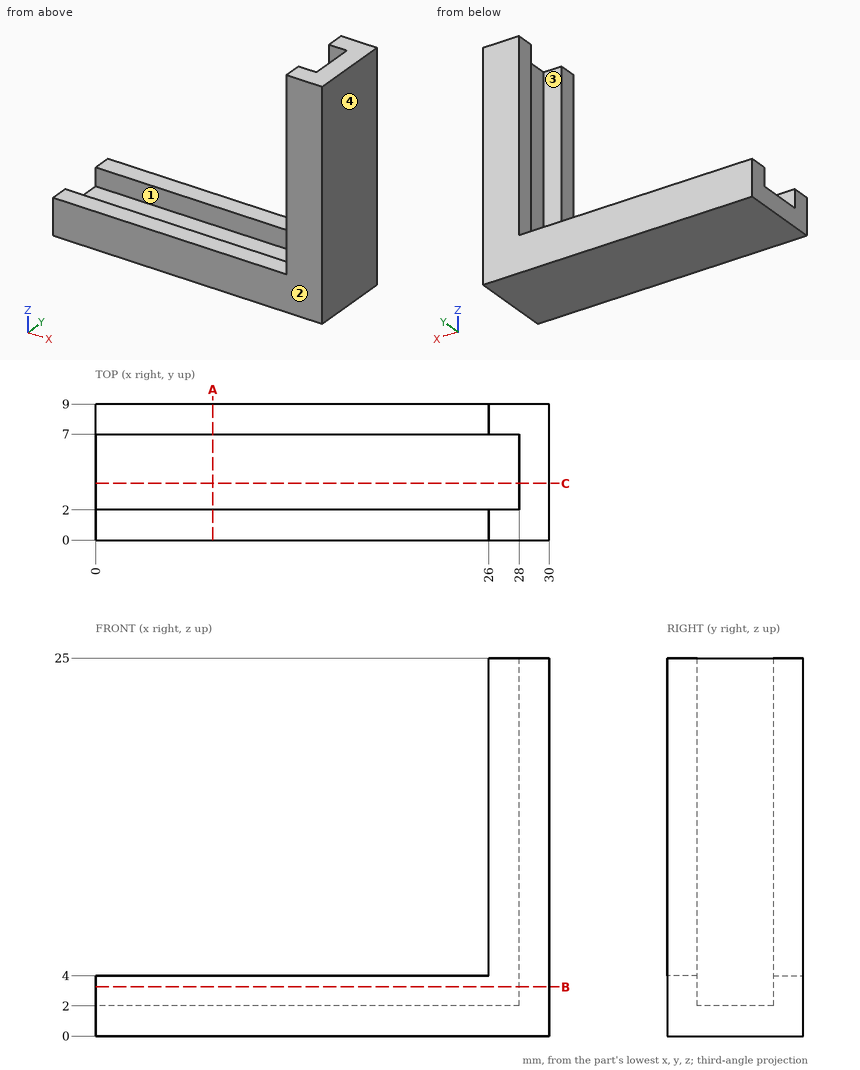
Could you check a few things on this drawing? It's one solid part, dimensions in mm from its lowest x, y, z. Coordinates: 2 decimals unless noted, no trailing zeros. Write each loop counter-clockwise with the first axis right and the second up, starting at its lowest first coordinate (ties: lowest second). Pieces come first, ordered by that corner, then holes. Notation, with made-up numbers: (78.5, -13.75) - (108.5, -13.75) arc R20 cw to (108.5, 24.25) - close; hole circle Ø4 at (3, -6.5). An arc over 180 degrees is marked (long way). Use one line per item in the form item = value.
1) Suppose I cut it at B-B, the plane z = 3.25. Write out the boundary of the cut face in (x, y), plus the area to 3 significant figures.
Solved:
outline = (0, 0) - (30, 0) - (30, 9) - (0, 9) - (0, 7) - (28, 7) - (28, 2) - (0, 2) - close
area = 130 mm2
2) Suppose I cut it at C-C, the plane y = 3.75. Write out the boundary of the cut face in (x, z).
Solved:
outline = (0, 0) - (30, 0) - (30, 25) - (28, 25) - (28, 2) - (0, 2) - close
3) I'm going to push flat-ended pins straight in: P1, Ø2, axis at x = 16.5, y = 1.5, coming from the +Z side; P2, Ø4, axis at x = 14.5, y = 2.5, coming from the -Z side; P3, Ø2.5, axis at y = 4, z = 15, coming from the -X side; P4, Ø2, axis at y = 1.5, z = 15.5, coming from the -X side. Where does each tip first touch, or does it pass through?
Solved:
P1 = 4
P2 = 0
P3 = 28
P4 = 26
4) Thinking about a two-plate mould opening in Y: for the marked faces 1, 2, 3 and 4, which applies, released by +Y, released by -Y, zero draft, split by the parting line, or undercut?
Solved:
face_1 = undercut
face_2 = released by -Y
face_3 = undercut
face_4 = zero draft
5) I need wall thicknesses on line 1 (Y direction, x = 2.75, z = 3.75); line 2 (Z direction, x = 8.25, y = 3.75); line 3 (X direction, y = 7.75, z = 13.5). Which ranges of each line are inside material? Lowest first, please.
Solved:
line_1 = 0 to 2, 7 to 9
line_2 = 0 to 2
line_3 = 26 to 30
6) Suppose I cut it at A-A, the plane x = 7.75. Write out the boundary of the cut face in (y, z).
Solved:
outline = (0, 0) - (9, 0) - (9, 4) - (7, 4) - (7, 2) - (2, 2) - (2, 4) - (0, 4) - close
